from build123d import *

# Parameters (mm, degrees)
F1_DEPTH = 7


with BuildPart() as f1:
    # F0 (on Top) → F1 (new body)
    with BuildSketch(Plane.XY):
        with BuildLine():
            ThreePointArc((16.89919, 52.010391), (10.231369, 36.021395), (7.956455, 18.847793))
            ThreePointArc((7.956455, 18.847793), (10.176788, 1.877889), (16.688307, -13.949545))
            ThreePointArc((16.688307, -13.949545), (21.916728, -19.257324), (29.127611, -21.13138))
            ThreePointArc((29.127611, -21.13138), (61.896865, -12.294717), (85.934267, 11.665958))
            ThreePointArc((85.934267, 11.665958), (87.916728, 18.847793), (85.934267, 26.029629))
            ThreePointArc((85.934267, 26.029629), (61.756138, 50.111193), (28.77906, 58.887066))
            ThreePointArc((28.77906, 58.887066), (21.938501, 57.00461), (16.89919, 52.010391))
        make_face()
        with BuildLine():
            ThreePointArc((32.916728, 18.847793), (34.267878, 24.12981), (37.9894, 28.114226))
            Line((37.9894, 28.114226), (36.465953, 30.752916))
            ThreePointArc((36.465953, 30.752916), (33.829532, 28.625544), (31.781291, 25.927185))
            Line((31.781291, 25.927185), (29.478451, 21.923404))
            Line((29.478451, 21.923404), (23.716056, 31.904166))
            ThreePointArc((23.716056, 31.904166), (29.182603, 30.890033), (34.612802, 32.083573))
            Line((34.612802, 32.083573), (33.066314, 34.641262))
            ThreePointArc((33.066314, 34.641262), (23.416728, 54.354835), (35.66439, 36.141262))
            Line((35.66439, 36.141262), (37.210878, 33.583573))
            ThreePointArc((37.210878, 33.583573), (40.948538, 37.671052), (42.808541, 42.888136))
            Line((42.808541, 42.888136), (48.493562, 32.869938))
            Line((48.493562, 32.869938), (43.874762, 32.873962))
            ThreePointArc((43.874762, 32.873962), (40.504687, 32.462287), (37.332809, 31.251476))
            Line((37.332809, 31.251476), (38.855426, 28.614226))
            ThreePointArc((38.855426, 28.614226), (49.416728, 28.374073), (54.905359, 19.347793))
            Line((54.905359, 19.347793), (57.866741, 19.347793))
            ThreePointArc((57.866741, 19.347793), (57.334459, 22.725785), (55.999117, 25.873962))
            Line((55.999117, 25.873962), (53.689716, 29.873962))
            Line((53.689716, 29.873962), (65.256474, 29.847793))
            ThreePointArc((65.256474, 29.847793), (61.668348, 25.628441), (59.997317, 20.347793))
            Line((59.997317, 20.347793), (63.019481, 20.347793))
            ThreePointArc((63.019481, 20.347793), (84.916728, 18.847793), (63.019481, 17.347793))
            Line((63.019481, 17.347793), (59.997317, 17.347793))
            ThreePointArc((59.997317, 17.347793), (61.668348, 12.067146), (65.256474, 7.847793))
            Line((65.256474, 7.847793), (53.696309, 7.870162))
            Line((53.696309, 7.870162), (55.999117, 11.873962))
            ThreePointArc((55.999117, 11.873962), (57.327231, 14.99697), (57.864871, 18.347793))
            Line((57.864871, 18.347793), (54.905359, 18.347793))
            ThreePointArc((54.905359, 18.347793), (49.416728, 9.321514), (38.855426, 9.08136))
            Line((38.855426, 9.08136), (37.355973, 6.484232))
            ThreePointArc((37.355973, 6.484232), (40.517398, 5.28249), (43.874762, 4.873962))
            Line((43.874762, 4.873962), (48.535531, 4.847793))
            Line((48.535531, 4.847793), (42.773135, -5.132969))
            ThreePointArc((42.773135, -5.132969), (40.913132, 0.084116), (37.175472, 4.171595))
            Line((37.175472, 4.171595), (35.66439, 1.554324))
            ThreePointArc((35.66439, 1.554324), (23.416728, -16.659248), (33.066314, 3.054324))
            Line((33.066314, 3.054324), (34.577396, 5.671595))
            ThreePointArc((34.577396, 5.671595), (29.168705, 6.864763), (23.720576, 5.867031))
            Line((23.720576, 5.867031), (29.441005, 15.873962))
            Line((29.441005, 15.873962), (31.750406, 11.873962))
            ThreePointArc((31.750406, 11.873962), (33.817227, 9.135071), (36.488181, 6.981173))
            Line((36.488181, 6.981173), (37.9894, 9.58136))
            ThreePointArc((37.9894, 9.58136), (34.267878, 13.565777), (32.916728, 18.847793))
        make_face(mode=Mode.SUBTRACT)
    extrude(amount=F1_DEPTH)


solid = f1.part
Could you check a few things on this model? Use its own coordinates, in mm. Round coordinates to 2 decimals unless told otherwise and drop trailing zeros. Write each loop counter-clockwise with the first axis right and the second up, starting at its lowest first coordinate (ties: lowest second). Pieces come first, ordered by that corner, then holes. Notation, with made-up numbers: (-39, 29.5) -> (4, 29.5) arc R15 cw to (4, 58.5) -> close; hole circle Ø6 at (74.25, -11.5). An arc over 180 degrees is marked (long way). Use a Markdown table: item, result.
1. Please list where these lines run through material, in increasing order: probe 1 along Y at (x, z) = (27, 2); probe 2 along Y at (x, z) = (37, 2.75); probe 3 along X at (y, z) = (10, 0.5).
Answer key:
| item | result |
|---|---|
| probe 1 | y = -21 to -17.96, 3.7 to 6.74, 11.6 to 26.22, 31.02 to 34, 55.66 to 58.75 |
| probe 2 | y = -20.63 to -14.59, 0.33 to 3.87, 7.87 to 10.29, 27.4 to 29.83, 33.93 to 37.37, 52.29 to 58.39 |
| probe 3 | x = 8.55 to 26.08, 33.05 to 37.38, 50.45 to 54.92, 63.07 to 67.38, 80.45 to 84.93 |
2. If we section it at D-D (y = -6.5): List the corners of the cut face in (x, z) for me.
Answer key:
| item | result |
|---|---|
| outline | (13.02, 0) -> (17.93, 0) -> (17.93, 7) -> (13.02, 7) -> close; (39.9, 0) -> (70.34, 0) -> (70.34, 7) -> (39.9, 7) -> close |
3. If we section it at A-A (x = 27.5): List the corners of the cut face in (y, z) for me, then the cut area to 3 significant figures.
Answer key:
| item | result |
|---|---|
| outline | (-21.06, 0) -> (-18.04, 0) -> (-18.04, 7) -> (-21.06, 7) -> close; (3.78, 0) -> (6.8, 0) -> (6.8, 7) -> (3.78, 7) -> close; (12.48, 0) -> (25.35, 0) -> (25.35, 7) -> (12.48, 7) -> close; (30.96, 0) -> (33.92, 0) -> (33.92, 7) -> (30.96, 7) -> close; (55.74, 0) -> (58.81, 0) -> (58.81, 7) -> (55.74, 7) -> close |
| area | 175 mm^2 |
4. We'd pull the mould along X, two halves only. Please class faces 1 (the face through (33.85, 33.345, 3.451)), 2 (the face through (22.026, 57.055, 3.451)): +X half, -X half, draft (parallel to the pull), parting line (faces both ways), or undercut.
Answer key:
| item | result |
|---|---|
| face 1 | undercut |
| face 2 | -X half |
5. If we section it at C-C (y = 39): List the corners of the cut face in (x, z) for me, then the cut area to 3 significant figures.
Answer key:
| item | result |
|---|---|
| outline | (11.11, 0) -> (19.59, 0) -> (19.59, 7) -> (11.11, 7) -> close; (38.25, 0) -> (41.65, 0) -> (41.65, 7) -> (38.25, 7) -> close; (45.01, 0) -> (76.08, 0) -> (76.08, 7) -> (45.01, 7) -> close |
| area | 301 mm^2 |
6. For pin 1 Ø2.5 at (x, z) = (61, 4) entering from -Y; pin 2 Ø1 at (x, z) = (31, 4) entering from +Y; pin 3 Ø1.5 at (x, z) = (62, 5) entering from +Y, each with a flat end and sliding along its axis, tell me the tip position at first contact or that it passes through.
Answer key:
| item | result |
|---|---|
| pin 1 | stops at y = -13.48 |
| pin 2 | stops at y = 58.87 |
| pin 3 | stops at y = 50.4 |
7. If we section it at B-B (x = 80): List the corners of the cut face in (y, z) for me.
Answer key:
| item | result |
|---|---|
| outline | (3.1, 0) -> (9.68, 0) -> (9.68, 7) -> (3.1, 7) -> close; (28.01, 0) -> (34.61, 0) -> (34.61, 7) -> (28.01, 7) -> close |
